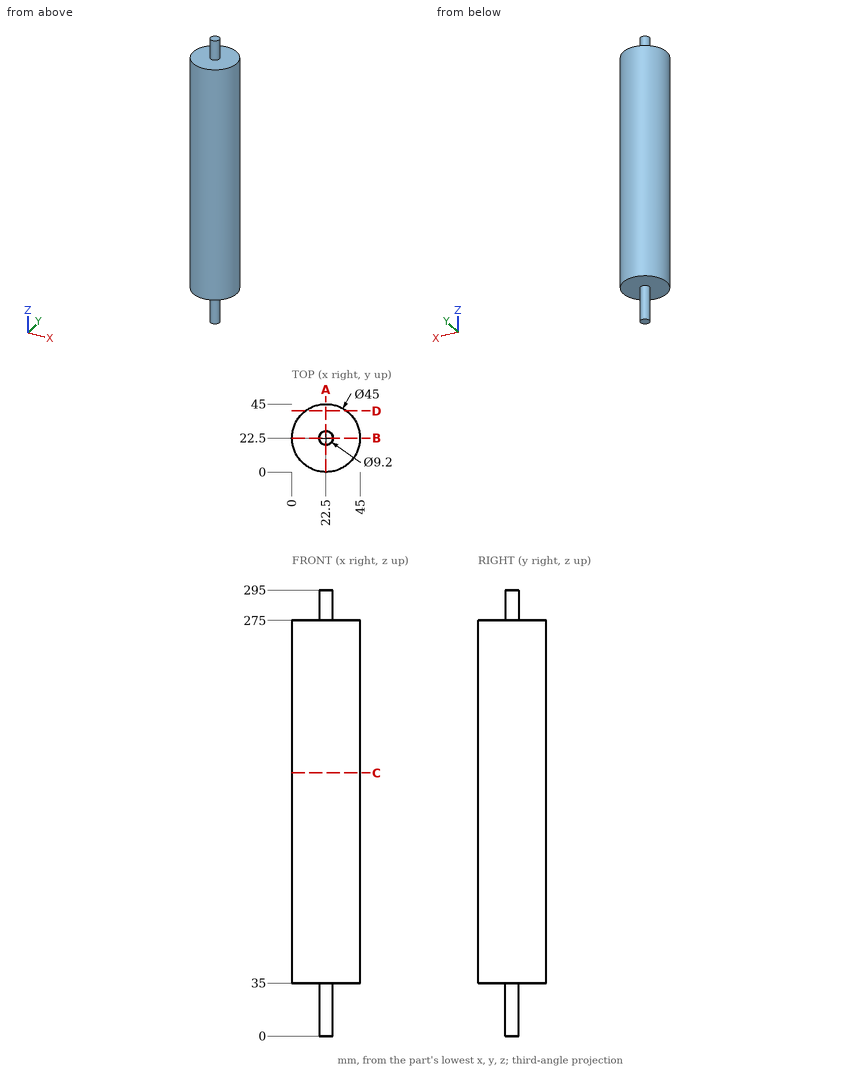
Source: three-view drawing plus pictorial views. Frame: mm from the lowest corner of the part. Give positions to 0.01 mm unless a question says otherwise; leave off trailing zeros. Loops run counter-clockwise (first coordinate to the right, second up) from the corner with the lowest first, then second, coordinate; pieces in that order, holes last. Notation, with made-up numbers: (-35, -6.75) -> (-20, -6.75) arc R25 cw to (-20, 26.25) -> close; hole circle Ø10 at (-26, 54.5). An arc over 180 degrees is marked (long way). Put each result on its own line as item: value. Start each with the question number.
1) Material intervals for probe 1 along Z at (x, y) = (35.5, 32); probe 2 along Y at (x, z) = (24, 143); probe 3 along Y at (x, z) = (38.5, 96), sorted ascending.
2) Cut plane D-D (y = 40.5). Return loops of the section in (x, z).
3) Contact query for flat-ended pins moving along their axis: P1, Ø2, axis at x = 13, y = 15.5, coming from the +Z side; P2, Ø3, axis at y = 31, z = 117.5, coming from the +X side; P3, Ø4, axis at x = 7, z = 221, coming from the +Y side. Output: stop coordinate, or through.
4) Cut plane C-C (z = 174). Return loops of the section in (x, y).
5) Cut plane A-A (x = 22.5). Return loops of the section in (y, z), then the cut area to 3 significant figures.
Results are:
1. probe 1: z = 35 to 275
1. probe 2: y = 0.05 to 44.95
1. probe 3: y = 6.68 to 38.32
2. outline: (9, 35) -> (36, 35) -> (36, 275) -> (9, 275) -> close
3. P1: stops at z = 275
3. P2: stops at x = 43.88
3. P3: stops at y = 40.5
4. outline: circle Ø45 at (22.5, 22.5)
5. outline: (0, 35) -> (17.9, 35) -> (17.9, 0) -> (27.1, 0) -> (27.1, 35) -> (45, 35) -> (45, 275) -> (27.1, 275) -> (27.1, 295) -> (17.9, 295) -> (17.9, 275) -> (0, 275) -> close
5. area: 11,300 mm2
